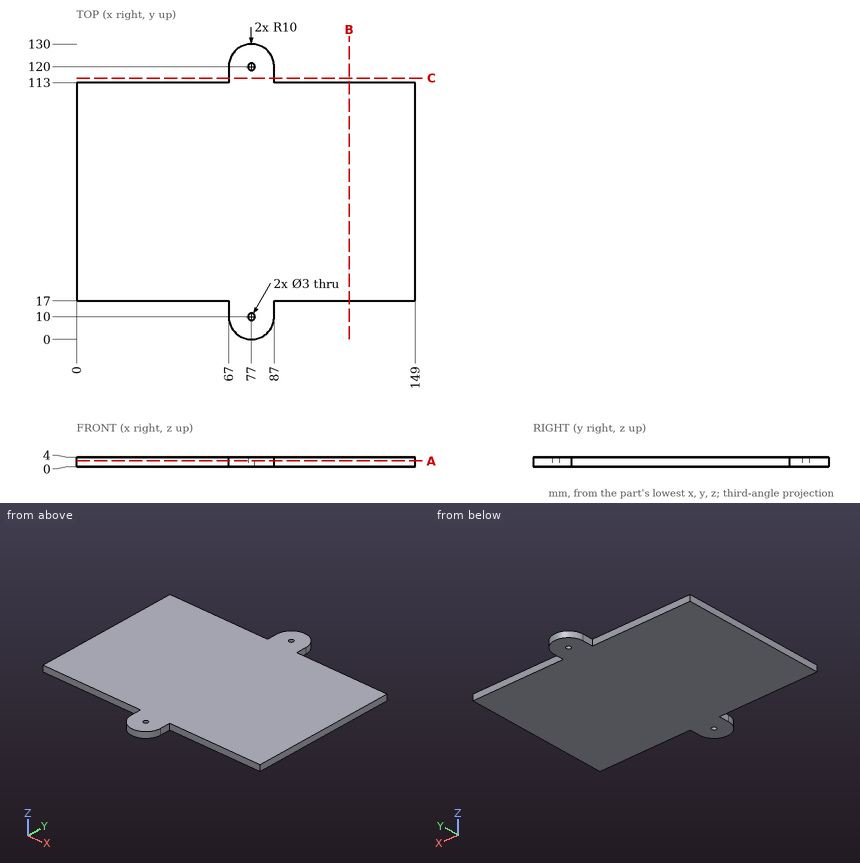
Source: three-view drawing plus pictorial views. Frame: mm from the lowest corner of the part. Round coordinates to 2 decimals unless told otherwise and drop trailing zeros. Loops run counter-clockwise (first coordinate to the right, second up) from the corner with the lowest first, then second, coordinate; pieces in that order, holes last.
Item 1: Line query: L1, parallel to Y at x = 77, z = 1.85; L2, parallel to Y at x = 76.5, z = 3.5; L3, parallel to X at y = 10, z = 1.95. Output: solid intervals per line, ascending.
Checked values:
L1: y = 0 to 8.5, 11.5 to 118.5, 121.5 to 130
L2: y = 0.01 to 8.59, 11.41 to 118.59, 121.41 to 129.99
L3: x = 67 to 75.5, 78.5 to 87
Item 2: Section B-B, the plane x = 120. Output: boundary loops of the cut face in (y, z).
Checked values:
outline: (17, 0) - (113, 0) - (113, 4) - (17, 4) - close
Item 3: Section A-A, the plane z = 2.45. Output: boundary loops of the cut face in (x, y).
Checked values:
outline: (0, 17) - (67, 17) - (67, 10) arc R10 ccw to (87, 10) - (87, 17) - (149, 17) - (149, 113) - (87, 113) - (87, 120) arc R10 ccw to (67, 120) - (67, 113) - (0, 113) - close; hole circle Ø3 at (77, 10); hole circle Ø3 at (77, 120)
Item 4: Contact query for flat-ended pins moving along their axis: P1, Ø1.2, axis at x = 117.5, z = 2, coming from the +Y side; P2, Ø1.8, axis at x = 77, y = 120, coming from the -Z side; P3, Ø2, axis at y = 13.5, z = 1, coming from the +X side; P4, Ø1.2, axis at y = 13.5, z = 2, coming from the -X side. Output: stop coordinate, or through.
Checked values:
P1: stops at y = 113
P2: passes through
P3: stops at x = 87
P4: stops at x = 67
Item 5: Section C-C, the plane y = 115. Output: boundary loops of the cut face in (x, z).
Checked values:
outline: (67, 0) - (87, 0) - (87, 4) - (67, 4) - close
